The listing builds one solid part. Answer for the finished solid, in the listing's coordinates (mm). Face numbers are marked on the shaded views. Round coordinates to 2 decimals unless told otherwise and drop trailing zeros. Write each loop counter-clockwise with the first axis right and the second up, starting at its lowest first coordinate (ties: lowest second). Pieces come first, ordered by that corner, then holes. Notation, with made-up numbers: (21.25, 8) - (27.25, 8) arc R23 ccw to (27.25, 29) - close; hole circle Ø4 at (83, 1.25). An arc over 180 degrees is marked (long way). Use a Markdown table: item, result. Add a question column.
1) Each of these flat-tipped pins is pushed along its axis until it touches: P1, Ø10, axis at x = 16, y = -101.5, coming from the +Z side; P2, Ø4, axis at x = -12, y = -116.5, coming from the -Z side; P3, Ø5, axis at x = -11.5, z = 4.5, coming from the +Y side. Where does it stop, or does it pass through?
2) A cutting plane is placed at B-B (x = 0). Give the vertices of the cut face in (y, z), then the cut area to 3 significant figures.
3) A cutting plane is placed at C-C (y = -26). Give the vertices of the cut face in (x, z), then the cut area to 3 significant figures.
4) A cutting plane is placed at A-A (z = 0). Give the vertices of the cut face in (x, y), then the cut area to 3 significant figures.
5) Determine the mould class of the marked faces 1, 2 and 3 for opening direction X: +X half, -X half, draft (parallel to the pull), parting line (faces both ways), or undercut.
6) Find the intervals of material crossed by probe 1 along Z at (x, y) = (0, -128); probe 2 along Z at (x, y) = (0, -47); probe 3 along X at (y, z) = (-48, 12.5), in increasing order. Write a range as from..to.
7) A cutting plane is placed at D-D (x = 7). Give the vertices of the cut face in (y, z) (3 decimals), then the cut area to 3 significant figures.
```python
from build123d import *

# Parameters (mm, degrees)
F0_R     = 20
F0_R_2   = 17.5
F1_DEPTH = 150
F2_W     = 2.265006
F2_H     = 14
F3_DEPTH = 50
F5_DEPTH = 42.001
F6_R     = 17.5
F6_R_2   = 11
F7_DEPTH = 50


with BuildPart() as f1:
    # F0 (on Front) → F1 (new body)
    with BuildSketch(Plane.XZ):
        Circle(F0_R)
        Circle(F0_R_2, mode=Mode.SUBTRACT)
    extrude(amount=F1_DEPTH)

    # F2 (on face) → F3 (join)
    with BuildSketch(Plane.XZ.offset(150)):
        with Locations((-19.867497, 0)):
            Rectangle(F2_W, F2_H)
        with Locations((19.867497, 0)):
            Rectangle(F2_W, F2_H)
    extrude(amount=-F3_DEPTH)

    # F4 (on face) → F5 (cut, through all)
    with BuildSketch(Plane(origin=(-21, 0, 0), x_dir=(0, -1, 0), z_dir=(-1, 0, 0))):
        with BuildLine():
            ThreePointArc((110, 2), (108, 0), (110, -2))
            Line((110, -2), (140, -2))
            ThreePointArc((140, -2), (142, 0), (140, 2))
            Line((140, 2), (110, 2))
        make_face()
    extrude(amount=-F5_DEPTH, mode=Mode.SUBTRACT)

    # F6 (on face) → F7 (join)
    with BuildSketch(Plane.XZ.offset(150)):
        Circle(F6_R)
        Circle(F6_R_2, mode=Mode.SUBTRACT)
    extrude(amount=-F7_DEPTH)


solid = f1.part
```
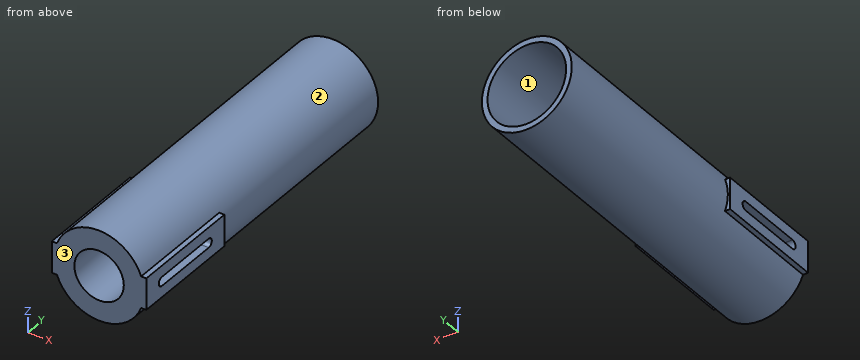
Entries:
| question | item | result |
|---|---|---|
| 1 | P1 | stops at z = 16.7 |
| 1 | P2 | stops at z = -17.32 |
| 1 | P3 | stops at y = -100 |
| 2 | outline | (-150, -20) - (0, -20) - (0, -17.5) - (-100, -17.5) - (-100, -11) - (-150, -11) - close; (-150, 11) - (-100, 11) - (-100, 17.5) - (0, 17.5) - (0, 20) - (-150, 20) - close |
| 2 | area | 1,400 mm² |
| 3 | outline | circle Ø40 at (0, 0); hole circle Ø35 at (0, 0) |
| 3 | area | 295 mm² |
| 4 | outline | (-21, -150) - (-11, -150) - (-11, -100) - (-17.5, -100) - (-17.5, 0) - (-20, 0) - (-20, -100) - (-21, -100) - (-21, -108) - (-17.5, -108) - (-17.5, -142) - (-21, -142) - close; (11, -150) - (21, -150) - (21, -142) - (17.5, -142) - (17.5, -108) - (21, -108) - (21, -100) - (20, -100) - (20, 0) - (17.5, 0) - (17.5, -100) - (11, -100) - close |
| 4 | area | 1,260 mm² |
| 5 | face 1 | undercut |
| 5 | face 2 | parting line |
| 5 | face 3 | draft |
| 6 | probe 1 | z = -20..-11, 11..20 |
| 6 | probe 2 | z = -20..-17.5, 17.5..20 |
| 6 | probe 3 | x = -15.61..-12.25, 12.25..15.61 |
| 7 | outline | (-150, -18.735) - (0, -18.735) - (0, -16.039) - (-100, -16.039) - (-100, -8.485) - (-150, -8.485) - close; (-150, 8.485) - (-100, 8.485) - (-100, 16.039) - (0, 16.039) - (0, 18.735) - (-150, 18.735) - close |
| 7 | area | 1,560 mm² |
